Here's the drawing with two shaded views (mm, measured from the low corner). I have some questions. A direction names the side the tool comes from. Coordinates: 2 decimals unless noted, no trailing zeros. Loops run counter-clockwise (first coordinate to the right, second up) from the corner with the lowest first, then second, coordinate; pieces in that order, holes last.
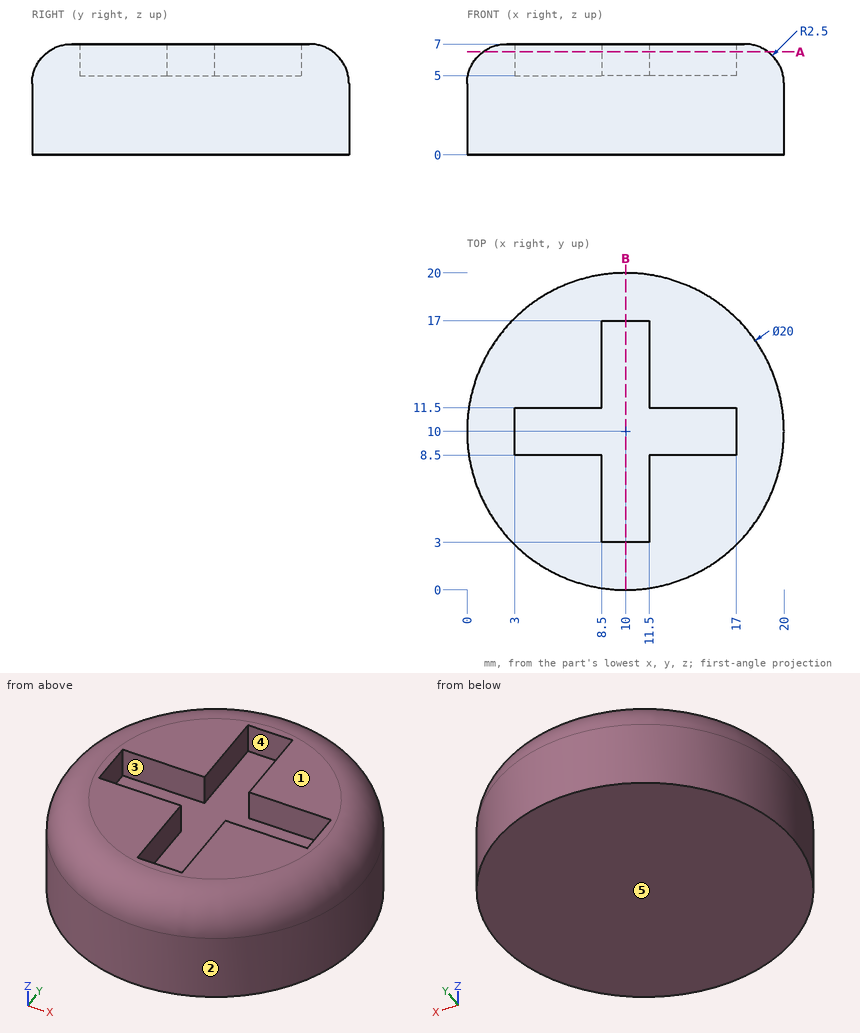
(1) If we mould it in two halves opening along Y, with no side actions, what happens to the marked faces 1, 2 and 3? For each: released by +Y, released by -Y, zero draft, split by the parting line, or undercut.
Check values:
face 1: zero draft
face 2: split by the parting line
face 3: undercut
(2) I want a section at B-B on x = 10. Write out the boundary of the cut face in (y, z).
Check values:
outline: (0, 0) - (20, 0) - (20, 4.5) arc R2.5 ccw to (17.5, 7) - (17, 7) - (17, 5) - (3, 5) - (3, 7) - (2.5, 7) arc R2.5 ccw to (0, 4.5) - close
(3) If I drill on probe 1 along X at (y, z) = (11, 6); probe 2 along Y at (x, z) = (3.25, 6.25); probe 3 along Z at (x, y) = (9.25, 15.25), over which ranges is the centre line in solid material (lowest first)?
Check values:
probe 1: x = 0.55 to 3, 17 to 19.45
probe 2: y = 3.62 to 8.5, 11.5 to 16.38
probe 3: z = 0 to 5
(4) Which directions (+Z, -Z, +X, -X, +Y, -Y) give clear straight access to the entire face, cutting with the end or side of a thin tool? Please do the marked faces 4 and 5.
Check values:
face 4: +Z
face 5: -Z, +X, -X, +Y, -Y
(5) I'm going to push flat-ended pins straight in: pin 1 (0.6 mm diameter, centred on x = 13.5, z = 6, fed in from +Y); pin 2 (0.6 mm diameter, centred on x = 10, z = 6, fed in from -Y); pin 3 (1.5 mm diameter, centred on x = 5, z = 5.5, fed in from +Y). Where does each tip first touch, or does it pass through?
Check values:
pin 1: stops at y = 19.07
pin 2: stops at y = 0.31
pin 3: stops at y = 18.92
(6) I want a section at A-A on z = 6.5. Write out the boundary of the cut face in (x, y), then the cut area to 3 significant figures.
Check values:
outline: circle Ø18 at (10, 10); hole (3, 8.5) - (8.5, 8.5) - (8.5, 3) - (11.5, 3) - (11.5, 8.5) - (17, 8.5) - (17, 11.5) - (11.5, 11.5) - (11.5, 17) - (8.5, 17) - (8.5, 11.5) - (3, 11.5) - close
area: 179 mm2
